```python
from build123d import *

# Parameters (mm, degrees)
SKETCH1_W           = 20
SKETCH1_H           = 10
BOSS_EXTRUDE1_DEPTH = 10
SKETCH2_W           = 16
SKETCH2_H           = 5
CUT_EXTRUDE1_DEPTH  = 11
SKETCH3_W           = 20
SKETCH3_H           = 15
BOSS_EXTRUDE2_DEPTH = 5
SKETCH4_W           = 14
SKETCH4_H           = 12
CUT_EXTRUDE2_DEPTH  = 4
CUT_EXTRUDE3_DEPTH  = 0.5
CUT_EXTRUDE4_DEPTH  = 21


with BuildPart() as part:
    # Sketch1 → Boss-Extrude1 (new body)
    with BuildSketch(Plane(origin=(0, 0, 0), x_dir=(1, 0, 0), z_dir=(0, 1, 0))):
        Rectangle(SKETCH1_W, SKETCH1_H)
    extrude(amount=BOSS_EXTRUDE1_DEPTH)

    # Sketch2 → Cut-Extrude1 (cut, through all)
    with BuildSketch(Plane(origin=(0, 10, 0), x_dir=(1, 0, 0), z_dir=(0, 1, 0))):
        Rectangle(SKETCH2_W, SKETCH2_H)
    extrude(amount=-CUT_EXTRUDE1_DEPTH, mode=Mode.SUBTRACT)

    # Sketch3 → Boss-Extrude2 (add)
    with BuildSketch(Plane.XY.offset(5)):
        with Locations((0, 7.5)):
            Rectangle(SKETCH3_W, SKETCH3_H)
    extrude(amount=BOSS_EXTRUDE2_DEPTH)

    # Sketch4 → Cut-Extrude2 (cut)
    with BuildSketch(Plane.XY.offset(10)):
        with Locations((0, 9)):
            Rectangle(SKETCH4_W, SKETCH4_H)
    extrude(amount=-CUT_EXTRUDE2_DEPTH, mode=Mode.SUBTRACT)

    # Sketch5 → Cut-Extrude3 (cut)
    with BuildSketch(Plane.XY.offset(10)):
        Polygon((-9, 15), (-9, 1), (0, 1), (9, 1), (9, 15), (8, 15), (8, 2), (0, 2), (-8, 2), (-8, 15), align=None)
    extrude(amount=-CUT_EXTRUDE3_DEPTH, mode=Mode.SUBTRACT)

    # Sketch7 → Cut-Extrude4 (cut, through all)
    with BuildSketch(Plane(origin=(10, 0, 0), x_dir=(0, 0, -1), z_dir=(1, 0, 0))):
        Polygon((5, 4.019237886), (-10, 0), (5, 0), align=None)
    extrude(amount=-CUT_EXTRUDE4_DEPTH, mode=Mode.SUBTRACT)


solid = part.part
```
For this review, take the finished solid that the model builds, in its own axes (mm). A direction names the side the tool comes from. Give positions to 0.01 mm unless a question says otherwise; leave off trailing zeros. Write each loop counter-clockwise with the first axis right and the second up, starting at its lowest first coordinate (ties: lowest second). Pieces come first, ordered by that corner, then holes. Notation, with made-up numbers: M 55.5,-8 L 84.5,-8 A17 ccw 84.5,15 Z; hole C 1.25,-36 d3. An arc over 180 degrees is marked long. Answer as CSV lines item,"result".
1. Consider section A-A, the plane y = 6. Write out the cut boundary in (x, z).
Findings:
outline,"M -10,-5 L 10,-5 L 10,10 L 9,10 L 9,9.5 L 8,9.5 L 8,10 L 7,10 L 7,6 L -7,6 L -7,10 L -8,10 L -8,9.5 L -9,9.5 L -9,10 L -10,10 Z; hole M -8,-2.5 L 8,-2.5 L 8,2.5 L -8,2.5 Z"
2. Wall thickness on line 1 (Z direction, x = -3, y = 9.25); line 2 (X direction, y = 4.75, z = 7.75); line 3 (X direction, y = 5.75, z = 1.25): over which ranges is each line inside the solid? List them lowest first.
Findings:
line 1,"z = -5 to -2.5, 2.5 to 6"
line 2,"x = -10 to -7, 7 to 10"
line 3,"x = -10 to -8, 8 to 10"
3. For pin 1 (7.5 mm diameter, centred on x = -0.5, y = 7.5, fed in from +Z); pin 2 (2 mm diameter, centred on x = 3, z = 8.5, fed in from +Y); pin 3 (2 mm diameter, centred on x = 7.5, z = 7, fed in from -Y), all flat-tipped, find the tip position at first contact; note any pin that passes through.
Findings:
pin 1,"stops at z = 6"
pin 2,"stops at y = 3"
pin 3,"stops at y = 0.54"
4. Consider section D-D, the plane x = 8.25. Write out the cut boundary in (y, z).
Findings:
outline,"M 0,10 L 4.02,-5 L 10,-5 L 10,5 L 15,5 L 15,9.5 L 1,9.5 L 1,10 Z"
5. Consider section C-C, the plane z = 1. Write out the cut boundary in (x, y), then the cut area to 3 significant figures.
Findings:
outline,"M -10,2.41 L -8,2.41 L -8,10 L -10,10 Z; M 8,2.41 L 10,2.41 L 10,10 L 8,10 Z"
area,"30.4 mm2"
6. Draft analysis for pull direction Y (two halves, no side actions). For faces 1 (the flat face through (0.14, 1.59, 4.06)), 2 (the flat face through (-10, 7, 4)), 3 (the flat face through (-1.4, 1.8, 9.5)), 4 (the flat face through (0, 10, -3)), state which applies: +Y half, -Y half, draft (parallel to the pull), parting line (faces both ways), or undercut.
Findings:
face 1,"-Y half"
face 2,"draft"
face 3,"undercut"
face 4,"+Y half"
7. For faces 5 (the flat face through (0, 13, 5)), 6 (the flat face through (0, 7, -2.5)), 7 (the flat face through (0, 3, 8)), 8 (the flat face through (-0.1, 15, 5.8)), list the 3-axis set-ups (+Z, -Z, +X, -X, +Y, -Y) from which the entire face can be reached by the end or side of a thin tool; tool diameter is ignored.
Findings:
face 5,"-Z, +X, -X, +Y"
face 6,"+Y, -Y"
face 7,"+Z, +Y"
face 8,"+Z, -Z, +X, -X, +Y"
8. Consider section B-B, the plane x = -6.5. Write out the cut boundary in (y, z).
Findings:
outline,"M 0,10 L 2.01,2.5 L 10,2.5 L 10,5 L 15,5 L 15,6 L 3,6 L 3,10 L 2,10 L 2,9.5 L 1,9.5 L 1,10 Z; M 3.35,-2.5 L 4.02,-5 L 10,-5 L 10,-2.5 Z"
